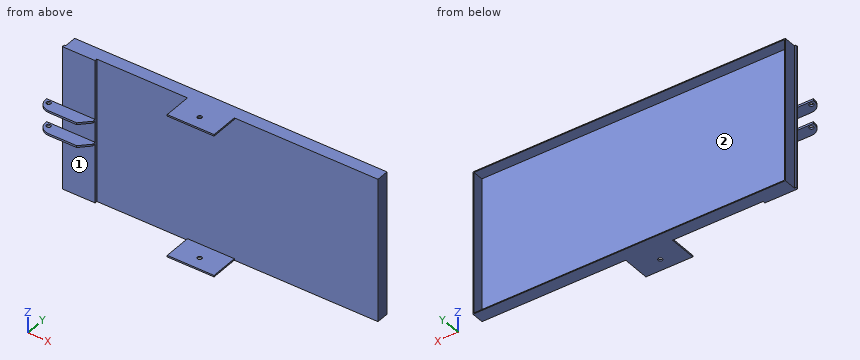
```python
from build123d import *

# Parameters (mm, degrees)
ESQUISSE2_W                  = 1000
ESQUISSE2_H                  = 460
BOSS_EXTRU_1_DEPTH           = 40
ESQUISSE3_W                  = 150
ESQUISSE3_H                  = 5
BOSS_EXTRU_2_DEPTH           = 90
ENL_V_MAT_EXTRU_1_REACH      = 1106.4
ESQUISSE4_R                  = 7
ESQUISSE5_W                  = 105
ESQUISSE5_H                  = 460
BOSS_EXTRU_3_DEPTH           = 8
ESQUISSE6_W                  = 155
ESQUISSE6_H                  = 6
BOSS_EXTRU_4_DEPTH           = 40
CHANFREIN1_SIZE              = 30
CONG_1_R                     = 35
ENL_V_MAT_EXTRU_2_REACH      = 1041.711
ESQUISSE7_R                  = 7
ESQUISSE8_W                  = 994
ESQUISSE8_H                  = 454
ENL_V_MAT_EXTRU_3_DEPTH      = 35
CHANFREIN1_OF_SYM_TRIE1_SIZE = 30
CONG_1_OF_SYM_TRIE1_R        = 35


with BuildPart() as part:
    # Esquisse2 → Boss.-Extru.1 (new body)
    with BuildSketch(Plane(origin=(0, 0, 0), x_dir=(1, 0, 0), z_dir=(0, 1, 0))):
        with Locations((500, 0)):
            Rectangle(ESQUISSE2_W, ESQUISSE2_H)
    extrude(amount=BOSS_EXTRU_1_DEPTH)

    # Esquisse3 → Boss.-Extru.2 (add)
    with BuildSketch(Plane.XZ):
        with Locations((465, 227.5)):
            Rectangle(ESQUISSE3_W, ESQUISSE3_H)
    boss_extru_2 = extrude(amount=BOSS_EXTRU_2_DEPTH)

    # Esquisse4 → Enlèv. mat.-Extru.1 (cut, up to next)
    with BuildSketch(Plane.XY.offset(230), mode=Mode.PRIVATE) as enl_v_mat_extru_1_sk1:
        with Locations((465, -50)):
            Circle(ESQUISSE4_R)
    enl_v_mat_extru_1_tool1 = extrude(enl_v_mat_extru_1_sk1.sketch, amount=-ENL_V_MAT_EXTRU_1_REACH, mode=Mode.PRIVATE) & part.part
    enl_v_mat_extru_1 = enl_v_mat_extru_1_tool1.solids().sort_by_distance((465, -50, 230))[0]
    add(enl_v_mat_extru_1, mode=Mode.SUBTRACT)

    # Esquisse5 → Boss.-Extru.3 (add)
    with BuildSketch(Plane.XZ):
        with Locations((47.5, 0)):
            Rectangle(ESQUISSE5_W, ESQUISSE5_H)
    extrude(amount=BOSS_EXTRU_3_DEPTH)

    # Esquisse6 → Boss.-Extru.4 (add)
    with BuildSketch(Plane.XZ.offset(8)):
        with Locations((22.5, 37)):
            Rectangle(ESQUISSE6_W, ESQUISSE6_H)
    boss_extru_4 = extrude(amount=BOSS_EXTRU_4_DEPTH)

    # Chanfrein1
    chanfrein1_edges = [part.edges().sort_by_distance(p)[0] for p in [
        (100, -48, 37),
    ]]
    chamfer(chanfrein1_edges, length=CHANFREIN1_SIZE)

    # Congé1
    cong_1_edges = [part.edges().sort_by_distance(p)[0] for p in [
        (-55, -48, 37),
    ]]
    fillet(cong_1_edges, radius=CONG_1_R)

    # Esquisse7 → Enlèv. mat.-Extru.2 (cut, up to next)
    with BuildSketch(Plane.XY.offset(40), mode=Mode.PRIVATE) as enl_v_mat_extru_2_sk1:
        with Locations((-40, -20)):
            Circle(ESQUISSE7_R)
    enl_v_mat_extru_2_tool1 = extrude(enl_v_mat_extru_2_sk1.sketch, amount=-ENL_V_MAT_EXTRU_2_REACH, mode=Mode.PRIVATE) & part.part
    enl_v_mat_extru_2 = enl_v_mat_extru_2_tool1.solids().sort_by_distance((-40, -20, 40))[0]
    add(enl_v_mat_extru_2, mode=Mode.SUBTRACT)

    # Esquisse8 → Enlèv. mat.-Extru.3 (cut)
    with BuildSketch(Plane(origin=(0, 40, 0), x_dir=(1, 0, 0), z_dir=(0, 1, 0))):
        with Locations((500, 0)):
            Rectangle(ESQUISSE8_W, ESQUISSE8_H)
    extrude(amount=-ENL_V_MAT_EXTRU_3_DEPTH, mode=Mode.SUBTRACT)

    # Symétrie1: Boss.-Extru.2, Enlèv. mat.-Extru.1, Boss.-Extru.4, Enlèv. mat.-Extru.2 across plane
    add(boss_extru_2.mirror(Plane(origin=(0, 0, 0), x_dir=(1, 0, 0), z_dir=(0, 0, -1))))
    add(enl_v_mat_extru_1.mirror(Plane(origin=(0, 0, 0), x_dir=(1, 0, 0), z_dir=(0, 0, -1))), mode=Mode.SUBTRACT)
    add(boss_extru_4.mirror(Plane(origin=(0, 0, 0), x_dir=(1, 0, 0), z_dir=(0, 0, -1))))
    add(enl_v_mat_extru_2.mirror(Plane(origin=(0, 0, 0), x_dir=(1, 0, 0), z_dir=(0, 0, -1))), mode=Mode.SUBTRACT)

    # Chanfrein1 of Symétrie1
    chanfrein1_of_sym_trie1_edges = [part.edges().sort_by_distance(p)[0] for p in [
        (100, -48, -37),
    ]]
    chamfer(chanfrein1_of_sym_trie1_edges, length=CHANFREIN1_OF_SYM_TRIE1_SIZE)

    # Congé1 of Symétrie1
    cong_1_of_sym_trie1_edges = [part.edges().sort_by_distance(p)[0] for p in [
        (-55, -48, -37),
    ]]
    fillet(cong_1_of_sym_trie1_edges, radius=CONG_1_OF_SYM_TRIE1_R)


solid = part.part
```
Work out the finished part from the listing and answer in its coordinate system (mm). Face numbers are marked on the shaded views. Give positions to 0.01 mm unless a question says otherwise; leave off trailing zeros. Order: outer loops, then holes, each group sorted by start corner. A loop starts at its lowest first (then second) coordinate and runs counter-clockwise, first axis right, second up.
1. Section B-B, the plane z = -16 is taken. Determine the outline of the cut face in (x, y), and give its area (3 significant figures).
Result sheet:
outline: (-5, -8) - (100, -8) - (100, 0) - (1000, 0) - (1000, 40) - (997, 40) - (997, 5) - (3, 5) - (3, 40) - (0, 40) - (0, 0) - (-5, 0) - close
area: 6,050 mm2
2. Each of these flat-tipped pins is pushed along its axis until it touches: P1, Ø6.5, axis at y = -2, z = -88.5, coming from the -X side; P2, Ø12, axis at x = 382, z = -57, coming from the -Y side; P3, Ø3, axis at x = -21.5, z = -36.5, coming from the +Y side; P4, Ø12.5, axis at x = 465, y = -50, coming from the +Z side. Where does it stop, or does it pass through?
Result sheet:
P1: stops at x = -5
P2: stops at y = 0
P3: stops at y = -8
P4: passes through
3. Straight lines are drawn through the part: L1, parallel to Z at x = 90, y = -23; L2, parallel to Z at x = 546, y = 22; L3, parallel to X at y = 14, z = 12. For each, find the intervals that lie inside material, in ascending order.
Result sheet:
L1: z = -40 to -34, 34 to 40
L2: z = -230 to -227, 227 to 230
L3: x = 0 to 3, 997 to 1000
4. Section A-A, the plane y = -69.5 is taken. Determine the outline of the cut face in (x, z).
Result sheet:
outline: (390, -230) - (540, -230) - (540, -225) - (390, -225) - close; (390, 225) - (540, 225) - (540, 230) - (390, 230) - close
5. The mould has two halves that part along X. Classify the marked faces 1 and 2: released by +X, released by -X, zero draft, split by the parting line, or undercut.
Result sheet:
face 1: zero draft
face 2: undercut
6. Section C-C, the plane x = 923 is taken. Determine the outline of the cut face in (y, z), and give its area (3 significant figures).
Result sheet:
outline: (0, -230) - (40, -230) - (40, -227) - (5, -227) - (5, 227) - (40, 227) - (40, 230) - (0, 230) - close
area: 2,510 mm2
